Check sheet for the drawn part. Datum: minimum x, y, z corner. Units: mm. A direction names the side the tool comes from. Round coordinates to 2 decimals unless told otherwise and drop trailing zeros. Write each loop counter-clockwise with the first axis right and the second up, starting at its lowest first coordinate (ties: lowest second). Pieces come first, ordered by that corner, then holes.
Item 1: Cross-section at A-A on x = 60. Enter the section's corners in (y, z).
Item 2: Cross-section at C-C on y = 21. Enter the section's corners in (x, z).
Item 3: Release check for a two-part mould opening along Z. For the marked faces 1, 2 and 3 record: +Z half, -Z half, draft (parallel to the pull), parting line (faces both ways), or undercut.
Item 4: Go/stop test with flat-tipped pins: pin 1 Ø1.5 at (x, z) = (90, 32) entering from -Y; pin 2 Ø8 at (x, z) = (14, 41) entering from +Y; pin 3 Ø1.5 at (y, z) = (220, 41.5) entering from +X. Record where each tip stops, or that it passes through.
Item 5: Cross-section at B-B on z = 72.5. Enter the section's corners in (x, y), plus the area to 3 significant figures.
Item 6: Material ranges on line 1 (Y direction, x = 102, z = 67); line 2 (Z direction, x = 30, y = 76.5); line 3 (Y direction, x = 80, z = 102), recorded low to high.
Item 7: Tool access check on the marked faces 4, 5 and 6. Record the directions out of +Z, -Z, +X, -X, +Y, -Y that give a thin tool (end or side, any length) a straight path to the whole face; none if there is none.
Item 8: Cross-section at D-D on x = 97. Enter the section's corners in (y, z).
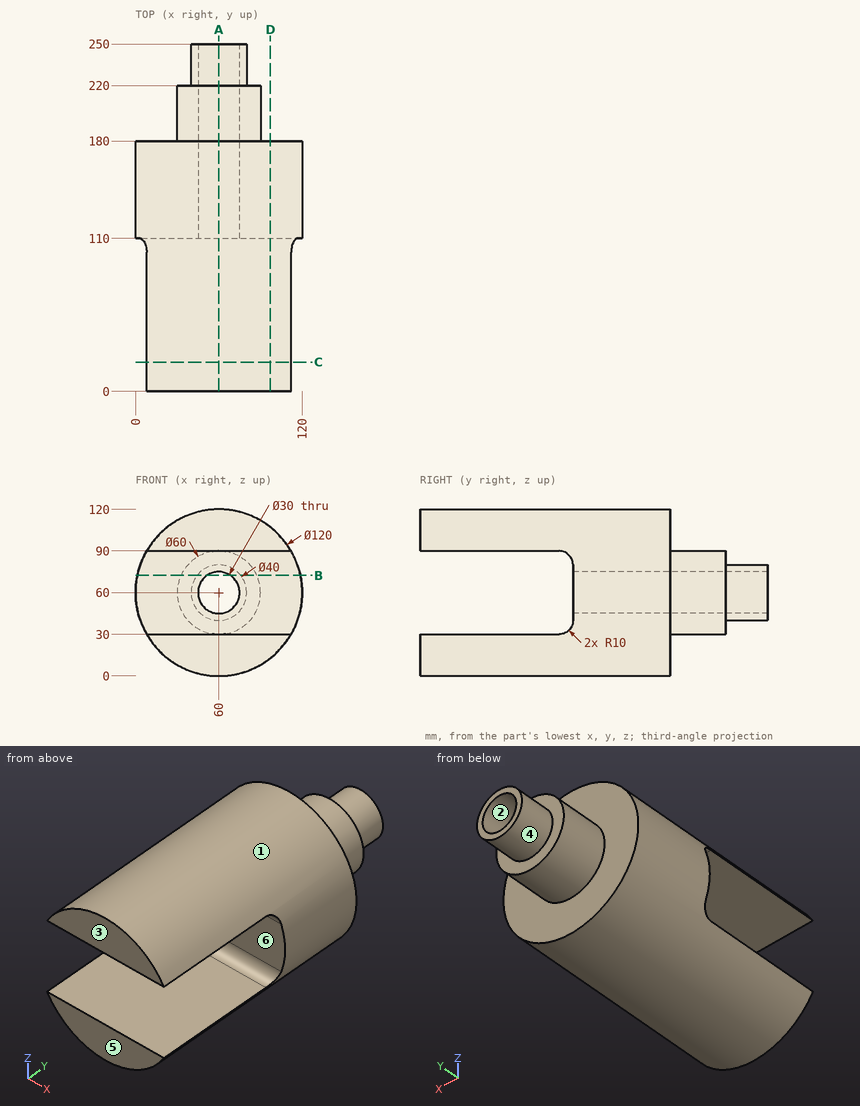
Response values:
1. outline: (0, 0) - (180, 0) - (180, 30) - (220, 30) - (220, 40) - (250, 40) - (250, 45) - (110, 45) - (110, 40) arc R10 cw to (100, 30) - (0, 30) - close; (0, 90) - (100, 90) arc R10 cw to (110, 80) - (110, 75) - (250, 75) - (250, 80) - (220, 80) - (220, 90) - (180, 90) - (180, 120) - (0, 120) - close
2. outline: (8.04, 30) arc R60 ccw to (111.96, 30) - close; (8.04, 90) - (111.96, 90) arc R60 ccw to start
3. face 1: parting line
3. face 2: undercut
3. face 3: draft
4. pin 1: stops at y = 104.84
4. pin 2: stops at y = 180
4. pin 3: stops at x = 84.19
5. outline: (1.32, 110) - (51.71, 110) - (51.71, 250) - (44.39, 250) - (44.39, 220) - (32.73, 220) - (32.73, 180) - (1.32, 180) - close; (68.29, 110) - (118.68, 110) - (118.68, 180) - (87.27, 180) - (87.27, 220) - (75.61, 220) - (75.61, 250) - (68.29, 250) - close
5. area: 9,010 mm2
6. line 1: y = 110 to 180
6. line 2: z = 8.04 to 30, 90 to 111.96
6. line 3: y = 0 to 180
7. face 4: +Y
7. face 5: +Z, -Z, +X, -X, -Y
7. face 6: +X, -X, -Y
8. outline: (0, 12.77) - (180, 12.77) - (180, 107.23) - (0, 107.23) - (0, 90) - (100, 90) arc R10 cw to (110, 80) - (110, 40) arc R10 cw to (100, 30) - (0, 30) - close
